Here's how the part is built. I have some questions about the finished solid (model axes, mm). Coordinates: 2 decimals unless noted, no trailing zeros. Order: outer loops, then holes, each group sorted by start corner. A loop starts at its lowest first (then second) coordinate and runs counter-clockwise, first axis right, second up. Notation, with made-up numbers: M -31,9 L -11,9 A9 ccw -11,19 Z; hole C 65.5,-17.5 d5. An arc over 180 degrees is marked long. Answer as CSV lines item,"result". Start each with the question number.
```python
from build123d import *

# Parameters (mm, degrees)
BOSS_EXTRUDE1_DEPTH = 2.5
FILLET1_R           = 1
BOSS_EXTRUDE2_DEPTH = 5


with BuildPart() as part:
    # Sketch1 → Boss-Extrude1 (new body)
    with BuildSketch(Plane.XY):
        Polygon((-2.5, 40), (-2.5, -30), (2.5, -30), (2.5, 40), (30, 40), (30, -40), (-30, -40), (-30, 40), align=None)
    extrude(amount=BOSS_EXTRUDE1_DEPTH)

    # Fillet1
    fillet1_edges = [part.edges().sort_by_distance(p)[0] for p in [
        (-2.5, 40, 1.25),
        (-2.5, -30, 1.25),
        (2.5, -30, 1.25),
        (2.5, 40, 1.25),
    ]]
    fillet(fillet1_edges, radius=FILLET1_R)

    # Sketch2 → Boss-Extrude2 (add)
    with BuildSketch(Plane(origin=(0, -30, 0), x_dir=(1, 0, 0), z_dir=(0, 1, 0))):
        with BuildLine():
            Line((-0.957859614, 0), (0.957859614, 0))
            ThreePointArc((0.957859614, 0), (1.5748, -1.25), (0.957859614, -2.5))
            Line((0.957859614, -2.5), (-0.957859614, -2.5))
            ThreePointArc((-0.957859614, -2.5), (-1.5748, -1.25), (-0.957859614, 0))
        make_face()
    extrude(amount=BOSS_EXTRUDE2_DEPTH)


solid = part.part
```
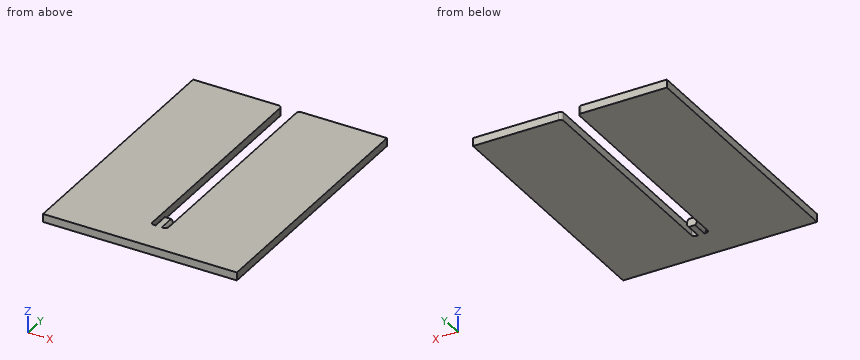
1) Suppose I cut it at A-A on y = 8. Please give me the cut outline in (x, z), plus the area to 4 significant figures.
2) Suppose I cut it at B-B on z = 1.25. Please give me the cut outline in (x, y), plus the area to 3 significant figures.
3) I need wall thicknesses on line 1 (X direction, y = -8, z = 1.1). Which ranges of the line are inside material? Lowest first, please. Write a range as [from, to].
4) Will this pin go through, and if not, where does the flat tip stop? pin 1 Ø0.8 at (x, z) = (-0.5, 1.5) entering from +Y.
Output:
1,outline,"M -30,0 L -2.5,0 L -2.5,2.5 L -30,2.5 Z; M 2.5,0 L 30,0 L 30,2.5 L 2.5,2.5 Z"
1,area,"137.5 mm²"
2,outline,"M -30,-40 L 30,-40 L 30,40 L 3.5,40 A1 ccw 2.5,39 L 2.5,-29 A1 cw 1.57,-30 L 1.57,-25 L -1.57,-25 L -1.57,-30 A1 cw -2.5,-29 L -2.5,39 A1 ccw -3.5,40 L -30,40 Z"
2,area,"4,470 mm²"
3,line 1,"[-30, -2.5], [2.5, 30]"
4,pin 1,"y = -25"
